from build123d import *

# Parameters (mm, degrees)
SKETCH1_R           = 7.8
BOSS_EXTRUDE1_DEPTH = 10
SKETCH2_R           = 1.55
CUT_EXTRUDE1_DEPTH  = 5
FILLET1_R           = 2


with BuildPart() as part:
    # Sketch1 → Boss-Extrude1 (new body)
    with BuildSketch(Plane.XY):
        with BuildLine():
            Line((-25, 0), (25, 0))
            Line((25, 0), (25, 5))
            Line((25, 5), (13.8, 5))
            Line((13.8, 5), (13.8, 18.2))
            ThreePointArc((13.8, 18.2), (0, 32), (-13.8, 18.2))
            Line((-13.8, 18.2), (-13.8, 5))
            Line((-13.8, 5), (-25, 5))
            Line((-25, 5), (-25, 0))
        make_face()
        with Locations((0, 18.2)):
            Circle(SKETCH1_R, mode=Mode.SUBTRACT)
    extrude(amount=-BOSS_EXTRUDE1_DEPTH)

    # Sketch2 → Cut-Extrude1 (cut)
    with BuildSketch(Plane(origin=(0, 5, 0), x_dir=(1, 0, 0), z_dir=(0, 1, 0))):
        with Locations((-19.4, 5)):
            Circle(SKETCH2_R)
    cut_extrude1 = extrude(amount=-CUT_EXTRUDE1_DEPTH, mode=Mode.SUBTRACT)

    # Mirror1: Cut-Extrude1 across plane
    add(cut_extrude1.mirror(Plane(origin=(0, 0, 0), x_dir=(0, 0, 1), z_dir=(1, 0, 0))), mode=Mode.SUBTRACT)

    # Fillet1
    fillet1_edges = [part.edges().sort_by_distance(p)[0] for p in [
        (-25, 5, -5),
        (-13.8, 5, -5),
        (13.8, 5, -5),
        (25, 5, -5),
    ]]
    fillet(fillet1_edges, radius=FILLET1_R)


solid = part.part
Model file for the job. Use its own axes, mm. A direction names the side the tool comes from. Give positions to 0.01 mm unless a question says otherwise; leave off trailing zeros. Order: outer loops, then holes, each group sorted by start corner. A loop starts at its lowest first (then second) coordinate and runs counter-clockwise, first axis right, second up. Notation, with made-up numbers: M 40,-17.75 L 82,-17.75 A13 cw 82,-13.75 Z; hole C 22.5,25.25 d10. An arc over 180 degrees is marked long. Write item = value, one per line.
Q1. Tool access for faces 1 (the flat face through (-13.8, 13, -5)), 2 (the cylindrical face through (17.968, 2.535, -4.406)), 3 (the flat face through (21.1, 5, -4.9)): list every direction of +Z, -Z, +X, -X, +Y, -Y with a clear straight run to the whole face (end or side of a thin tool).
Derived:
face_1 = +Z, -Z, -X, +Y
face_2 = +Y, -Y
face_3 = +Z, -Z, +X, +Y
Q2. Drill centre lines: line 1 (X direction, y = 2.8, z = -5); line 2 (Z direction, x = 19.4, y = 1.6); line 3 (Y direction, x = 0, z = -4). Where is each one in solid material? Low to high. Write a range as [from, to].
Derived:
line_1 = [-25, -20.95], [-17.85, 17.85], [20.95, 25]
line_2 = [-10, -6.55], [-3.45, 0]
line_3 = [0, 10.4], [26, 32]
Q3. Cut at A-A, the plane z = -5. List the corners of the cut face in (x, y), then the cut area to 3 significant figures.
Derived:
outline = M -25,0 L -20.95,0 L -20.95,5 L -23,5 A2 ccw -25,3 Z; M -17.85,0 L 17.85,0 L 17.85,5 L 15.8,5 A2 cw 13.8,7 L 13.8,18.2 A13.8 ccw -13.8,18.2 L -13.8,7 A2 cw -15.8,5 L -17.85,5 Z; M 20.95,0 L 25,0 L 25,3 A2 ccw 23,5 L 20.95,5 Z; hole C 0,18.2 d15.6
area = 691 mm2
Q4. Cut at D-D, the plane z = -1.5. List the corners of the cut face in (x, y).
Derived:
outline = M -25,0 L 25,0 L 25,3 A2 ccw 23,5 L 15.8,5 A2 cw 13.8,7 L 13.8,18.2 A13.8 ccw -13.8,18.2 L -13.8,7 A2 cw -15.8,5 L -23,5 A2 ccw -25,3 Z; hole C 0,18.2 d15.6
Q5. Cut at B-B, the plane x = 19.4. List the corners of the cut face in (y, z), then the cut area to 3 significant figures.
Derived:
outline = M 0,-10 L 5,-10 L 5,-6.55 L 0,-6.55 Z; M 0,-3.45 L 5,-3.45 L 5,0 L 0,0 Z
area = 34.5 mm2
Q6. Two-plate mould, pull along X, no slides. Class faces 4 (the cylindrical face through (-5.75, 23.47, -4.93)), 5 (the flat face through (0, 9, 0)), 6 (the cylindrical face through (24.43, 4.4, -5.07)): pulls with the +X half, pulls with the -X half, needs draft (parallel to the pull), parting line crosses it, or undercut.
Derived:
face_4 = undercut
face_5 = needs draft
face_6 = pulls with the +X half
Q7. Flat gauge pins, fed straight in: pin 1 (1.5 mm diameter, centred on y = 11, z = -2.5, fed in from -X); pin 2 (3.5 mm diameter, centred on x = 18.5, z = -4.5, fed in from +Y); pin 3 (2 mm diameter, centred on x = -12, z = -4, fed in from +Y). Where does each tip first touch, or does it go through?
Derived:
pin_1 = -13.8
pin_2 = 5
pin_3 = 26.53
Q8. Cut at C-C, the plane y = 17. List the corners of the cut face in (x, z).
Derived:
outline = M -13.8,-10 L -7.71,-10 L -7.71,0 L -13.8,0 Z; M 7.71,-10 L 13.8,-10 L 13.8,0 L 7.71,0 Z
